from build123d import *

# Parameters (mm, degrees)
SKETCH2_R            = 16.75
BOSS_EXTRUDE2_DEPTH  = 4
SKETCH1_R            = 14.75
CUT_EXTRUDE1_DEPTH   = 20
FILLET1_R            = 1
FILLET1_OF_MIRROR5_R = 1


with BuildPart() as part:
    # Sketch2 → Boss-Extrude2 (new body)
    with BuildSketch(Plane.XY):
        Circle(SKETCH2_R)
    boss_extrude2 = extrude(amount=BOSS_EXTRUDE2_DEPTH)

    # Sketch1 → Cut-Extrude1 (cut)
    with BuildSketch(Plane.XY):
        Circle(SKETCH1_R)
    cut_extrude1 = extrude(amount=CUT_EXTRUDE1_DEPTH, mode=Mode.SUBTRACT)

    # Fillet1
    fillet1_edges = [part.edges().sort_by_distance(p)[0] for p in [
        (-14.75, 0, 4),
    ]]
    fillet(fillet1_edges, radius=FILLET1_R)

    # Mirror5: Boss-Extrude2, Cut-Extrude1 across plane
    add(boss_extrude2.mirror(Plane(origin=(16.25, 0, 0), x_dir=(0, 0, 1), z_dir=(1, 0, 0))))
    add(cut_extrude1.mirror(Plane(origin=(16.25, 0, 0), x_dir=(0, 0, 1), z_dir=(1, 0, 0))), mode=Mode.SUBTRACT)

    # Fillet1 of Mirror5
    fillet1_of_mirror5_edges = [part.edges().sort_by_distance(p)[0] for p in [
        (47.25, 0, 4),
    ]]
    fillet(fillet1_of_mirror5_edges, radius=FILLET1_OF_MIRROR5_R)


solid = part.part
Could you check a few things on this model? Use its own coordinates, in mm. Give positions to 0.01 mm unless a question says otherwise; leave off trailing zeros. Write each loop counter-clockwise with the first axis right and the second up, starting at its lowest first coordinate (ties: lowest second). Pieces come first, ordered by that corner, then holes. Notation, with made-up numbers: (49, 56.5) -> (64, 56.5) arc R19 ccw to (64, 65.5) -> close; hole circle Ø5 at (86, -26). An arc over 180 degrees is marked (long way). Answer as a JSON object with one key per item and string values.
Q1. We'd pull the mould along X, two halves only. Please class faces 1 (the cylindrical face through (49.236, 0.679, 1.972)), 2 (the flat face through (16, 0, 4)): released by +X, released by -X, zero draft, split by the parting line, or undercut.
Taken from the geometry:
{"face 1": "undercut", "face 2": "zero draft"}
Q2. Please list where these lines run through material, in increasing order: L1, parallel to Y at x = 32.5, z = 1.85; L2, parallel to X at y = -10, z = 3; L3, parallel to X at y = 2, z = 3.25.
Taken from the geometry:
{"L1": "y = -16.75 to -14.75, 14.75 to 16.75", "L2": "x = -13.44 to -10.84, 10.84 to 13.44, 19.06 to 21.66, 43.34 to 45.94", "L3": "x = -16.63 to -14.65, 14.65 to 17.85, 47.15 to 49.13"}
Q3. Suppose I cut it at B-B on x = 32.5. Write out the boundary of the cut face in (y, z).
Taken from the geometry:
{"outline": "(-16.75, 0) -> (-14.75, 0) -> (-14.75, 3) arc R1 ccw to (-15.75, 4) -> (-16.75, 4) -> close; (14.75, 0) -> (16.75, 0) -> (16.75, 4) -> (15.75, 4) arc R1 ccw to (14.75, 3) -> close"}
Q4. Will this pin go through, and if not, where does the flat tip stop? pin 1 Ø8 at (x, y) = (24.5, 12.5) entering from -Z.
Taken from the geometry:
{"pin 1": "stops at z = 0"}
Q5. Suppose I cut it at A-A on y = 0. Write out the boundary of the cut face in (x, z), then the cut area to 3 significant figures.
Taken from the geometry:
{"outline": "(-16.75, 0) -> (-14.75, 0) -> (-14.75, 3) arc R1 ccw to (-15.75, 4) -> (-16.75, 4) -> close; (14.75, 0) -> (17.75, 0) -> (17.75, 3) arc R1 ccw to (16.75, 4) -> (15.75, 4) arc R1 ccw to (14.75, 3) -> close; (47.25, 0) -> (49.25, 0) -> (49.25, 4) -> (48.25, 4) arc R1 ccw to (47.25, 3) -> close", "area": "27.1 mm²"}
